For this review, take the finished solid that the model builds, in its own axes (mm). A direction names the side the tool comes from. Coordinates: 2 decimals unless noted, no trailing zeros. Write each loop counter-clockwise with the first axis right and the second up, starting at its lowest first coordinate (ties: lowest second). Pieces come first, ordered by that corner, then holes.
Autodesk Inventor part; units mm, degrees
ref_plane "YZ Plane" through (0, 0, 0) normal (1, 0, 0) x (0, 1, 0)
ref_plane "XZ Plane" through (0, 0, 0) normal (0, 1, 0) x (-1, 0, 0)
ref_plane "XY Plane" through (0, 0, 0) normal (0, 0, 1) x (1, 0, 0)
sketch "Sketch1" plane through (0, 0, 0) normal (0, 0, 1) x (1, 0, 0)
  circle A0 centre (0, 0) radius 3.6957
  dimension "d0" = 7.3914
extrude "Extrusion1" add sketch "Sketch1" along normal blind 4.0386
sketch "Sketch2" plane through (0, 0, 4.0386) normal (0, 0, 1) x (1, 0, 0)
  circle A0 centre (0, 0) radius 3.6957
  circle A1 centre (0, 0) radius 2.4003
  dimension "d3" = 1.2954
extrude "Extrusion2" cut sketch "Sketch2" against normal blind 2.7432 contours A1
sketch "Sketch3" plane through (0, 0, 0) normal (0, 0, -1) x (-1, 0, 0)
  circle A0 centre (0, 0) radius 3.6957
  circle A1 centre (0, 0) radius 2.1717
  dimension "d6" = 1.524
extrude "Extrusion3" cut sketch "Sketch3" against normal blind 1.0668 contours A1
sketch "Sketch4" plane through (0, 0, 1.2954) normal (0, 0, 1) x (1, 0, 0)
  circle A0 centre (0, 0) radius 2.4003
  circle A1 centre (0, 0) radius 1.4478
  dimension "d9" = 2.8956
extrude "Extrusion4" cut sketch "Sketch4" against normal through all contours A1
ref_plane "Work Plane1" through (0, 0, 0.5334) normal (0, 0, -1) x (-1, 0, 0)
sketch "Sketch5" plane through (0, 0, 0.5334) normal (0, 0, -1) x (-1, 0, 0)
  circle A0 centre (0, 0) radius 3.6957
  line L0 (-2.6602, 2.5654) -> (-16.3171, 1.6256)
  line L1 (-2.6602, -2.5654) -> (-16.3171, -1.6256)
  arc A1 (-16.3171, 1.6256) -> (-16.3171, -1.6256) centre (-16.2052, 0) ccw
  circle A2 centre (0, 0) radius 2.4003
  line L2 (2.6602, 2.5654) -> (16.3171, 1.6256)
  arc A3 (16.3171, -1.6256) -> (16.3171, 1.6256) centre (16.2052, 0) ccw
  line L3 (2.6602, -2.5654) -> (16.3171, -1.6256)
  dimension "d12" = 5.1308
  dimension "d15" = 16.2052
  dimension "d28" = 360
  dimension "d35" = 3.2512
extrude "Extrusion5" add sketch "Sketch5" along normal mid plane 1.0668 contours A0 L1 A1 L0
sketch "Sketch6" plane through (0, 0, 0) normal (0, 0, -1) x (-1, 0, 0)
  circle A0 centre (0, 0) radius 2.1717
  circle A1 centre (-4.4831, 0) radius 0.508
  dimension "d36" = 1.8034
  dimension "d37" = 1.016
extrude "Extrusion6" cut sketch "Sketch6" against normal through all contours A1
pattern_linear "Rectangular Pattern1" count 7 spacing 1.8288 along (1, 0, 0) of "Extrusion6"
properties part number "singleSideCutoff"
1) For L1, parallel to Y at x = 0, z = 2.45; L2, parallel to Z at x = 10, y = 1.75; L3, parallel to X at y = 0.25, z = 1.7, list the stretches that pass through material, from the lowest coordinate up.
2) Consider section A-A (x = 0). Give the boundary of the cut face in (y, z).
3) Clearance check with flat-ended pins moving along their axes: P1, Ø4, axis at x = 0, y = 0, coming from the -Z side; P2, Ø2.5, axis at x = 11.5, y = -0.5, coming from the +Z side; P3, Ø1.5, axis at x = 12, z = 1.5, coming from the +Y side; P4, Ø0.6, axis at x = 9.97, y = 0, coming from the +Z side. State where each tip first meets the part, or that it passes through.
4) Consider section B-B (y = -1). Give the boundary of the cut face in (x, z).
5) The part is to be moulded in two halves that separate along X. For faces 1 (the face through (17.834, -0.034, 0.541)), 2 (the face through (0, -2, 1.295)), 3 (the face through (15.963, 0.022, 0.526)), 4 (the face through (10, -1, 1.067)), say which applies: pulls with the +X half, pulls with the -X half, needs draft (parallel to the pull), parting line crosses it, or undercut.
6) Tool access review of faces 5 (the face through (-3.692, -0.162, 1.991)), 6 (the face through (0.47, -2.12, 0.53)), 7 (the face through (7, 0, 0)): name each direction out of +Z, -Z, +X, -X, +Y, -Y from which nothing blocks a thin tool from reaching the whole face with its end or side.
7) Consider section C-C (y = 0). Count the separate pieces of the cut face and the enclosed holes in it, then the cut area to 3 significant figures.
8) Consider section D-D (z = 1.8). Give the boundary of the cut face in (x, y), then the cut area to 3 significant figures.
Results:
1. L1: y = -3.7 to -2.4, 2.4 to 3.7
1. L2: z = 0 to 1.07
1. L3: x = -3.69 to -2.39, 2.39 to 3.69
2. outline: (-3.7, 0) - (-2.17, 0) - (-2.17, 1.07) - (-1.45, 1.07) - (-1.45, 1.3) - (-2.4, 1.3) - (-2.4, 4.04) - (-3.7, 4.04) - close; (1.45, 1.07) - (2.17, 1.07) - (2.17, 0) - (3.7, 0) - (3.7, 4.04) - (2.4, 4.04) - (2.4, 1.3) - (1.45, 1.3) - close
3. P1: stops at z = 1.07
3. P2: stops at z = 1.07
3. P3: stops at y = 1.96
3. P4: passes through
4. outline: (-3.56, 0) - (-1.93, 0) - (-1.93, 1.07) - (-1.05, 1.07) - (-1.05, 1.3) - (-2.18, 1.3) - (-2.18, 4.04) - (-3.56, 4.04) - close; (1.05, 1.07) - (1.93, 1.07) - (1.93, 0) - (17.49, 0) - (17.49, 1.07) - (3.56, 1.07) - (3.56, 4.04) - (2.18, 4.04) - (2.18, 1.3) - (1.05, 1.3) - close
5. face 1: pulls with the +X half
5. face 2: undercut
5. face 3: undercut
5. face 4: needs draft
6. face 5: +Z
6. face 6: -Z
6. face 7: -Z, +X, -X, +Y, -Y
7. separate pieces: 9
7. enclosed holes: 0
7. area: 18.9 mm2
8. outline: circle Ø7.39 at (0, 0); hole circle Ø4.8 at (0, 0)
8. area: 24.8 mm2
